Could you check a few things on this model? Use its own coordinates, in mm. Face numbers are marked on the shaded views. A direction names the side the tool comes from. Coordinates: 2 decimals unless noted, no trailing zeros. Loops run counter-clockwise (first coordinate to the right, second up) from the corner with the lowest first, then second, coordinate; pieces in that order, holes last. Notation, with made-up numbers: (-36, 89) - (9, 89) arc R17 cw to (9, 112) - close; hole circle Ø4 at (32, -1). An arc over 180 degrees is marked (long way). One line per question, with ' | ' between items. Start each with the question number.
1. Which directions (+Z, -Z, +X, -X, +Y, -Y) give clear straight access to the entire face, cutting with the end or side of a thin tool? Please do the marked faces 1 and 2.
2. I want a section at B-B, the plane z = -181. Write out the boundary of the cut face in (x, y), then the cut area to 3 significant figures.
3. We'd pull the mould along X, two halves only. Please class the marked faces 3, 4, 5 and 6: pulls with the +X half, pulls with the -X half, needs draft (parallel to the pull), parting line crosses it, or undercut.
4. I'm going to push flat-ended pins straight in: P1, Ø6, axis at x = -180, y = -168, coming from the -Z side; P2, Ø3, axis at x = -145.5, z = -154, coming from the +Y side; P3, Ø4, axis at x = 26, z = 24.5, coming from the -Y side; P4, Ø8, axis at x = 213.5, y = -84.5, coming from the +Z side. Where does each tip first touch, or does it pass through?
5. I want a section at C-C, the plane x = 220.5. Write out the boundary of the cut face in (y, z), then the cut area to 3 significant figures.
6. Please list where these lines run through material, in increasing order: L1, parallel to Y at x = 174.5, z = 44.5; L2, parallel to Z at x = -212, y = -146; L3, parallel to X at y = -142, z = 109. Write a range as [from, to].
7. I want a section at A-A, the plane y = -101. Write out the boundary of the cut face in (x, z).
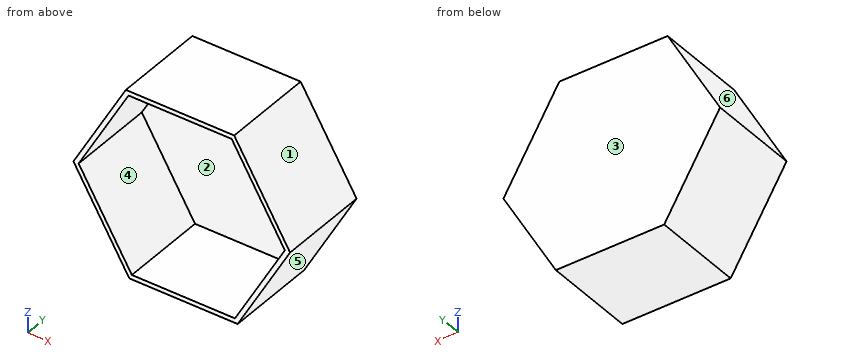
from build123d import *

# Parameters (mm, degrees)
F1_DEPTH = 254
F2_T     = -12.7


with BuildPart() as f1:
    # F0 (on Front) → F1 (new body)
    with BuildSketch(Plane.XZ):
        Polygon((-157.257091, 261.100072), (-304.74784, -5.6386), (-147.490749, -266.738671), (157.257091, -261.100072), (304.74784, 5.6386), (147.490749, 266.738671), align=None)
    extrude(amount=F1_DEPTH)

    # F2
    f2_openings = [f1.faces().sort_by_distance(p)[0] for p in [
        (0, -254, 0),
    ]]
    offset(amount=F2_T, openings=f2_openings)


with BuildPart() as f3_1:
    # F3: copy of F1
    add(f1.part.moved(Location((557.77382, 0, 309.68302))))


solid = f1.part
Results are:
1) face 1: +Z, +X, +Y, -Y | face 2: -Y
2) outline: (-199.13, -254) - (-184.3, -254) - (-184.3, -12.7) - (187.04, -12.7) - (187.04, -254) - (201.55, -254) - (201.55, 0) - (-199.13, 0) - close | area: 12,200 mm2
3) face 3: needs draft | face 4: undercut | face 5: pulls with the +X half | face 6: pulls with the -X half
4) P1: stops at z = -217.74 | P2: stops at y = 0 | P3: stops at y = -12.7 | P4: stops at z = 163.78
5) outline: (-254, -146.72) - (0, -146.72) - (0, 145.52) - (-254, 145.52) - (-254, 120.9) - (-12.7, 120.9) - (-12.7, -120.48) - (-254, -120.48) - close | area: 16,000 mm2
6) L1: y = [-12.7, 0] | L2: z = [-159.63, -135.02], [135.85, 162.1] | L3: x = [-241.36, -226.85], [227.67, 242.49]
7) outline: (-304.75, -5.64) - (-147.49, -266.74) - (157.26, -261.1) - (304.75, 5.64) - (147.49, 266.74) - (-157.26, 261.1) - close; hole (-290.09, -5.37) - (-140.39, -253.91) - (149.69, -248.54) - (290.09, 5.37) - (140.39, 253.91) - (-149.69, 248.54) - close
